Design review of the part built by this model. Coordinates are the model's own, in mm. A direction names the side the tool comes from. Coordinates: 2 decimals unless noted, no trailing zeros. Order: outer loops, then holes, each group sorted by start corner. A loop starts at its lowest first (then second) coordinate and runs counter-clockwise, first axis right, second up. Notation, with made-up numbers: M 89,55.25 L 122,55.25 A21 cw 122,83.25 Z; hole C -13,82.5 d10. An arc over 180 degrees is marked long. Use CSV: the item, a comma, the result in double quotes.
Autodesk Inventor part; units mm, degrees
ref_plane "YZ Plane" through (0, 0, 0) normal (1, 0, 0) x (0, 1, 0)
ref_plane "XZ Plane" through (0, 0, 0) normal (0, 1, 0) x (-1, 0, 0)
ref_plane "XY Plane" through (0, 0, 0) normal (0, 0, 1) x (1, 0, 0)
sketch "スケッチ1" plane through (0, 0, 0) normal (0, 0, 1) x (1, 0, 0)
  line L0 (0, 0) -> (65, 0)
  line L1 (65, 0) -> (65, 56)
  line L2 (65, 56) -> (0, 56)
  line L3 (0, 56) -> (0, 0)
  dimension "d0" = 56
  dimension "d1" = 65
extrude "押し出し1" add sketch "スケッチ1" along normal blind 1.5
sketch "スケッチ2" plane through (0, 0, 1.5) normal (0, 0, 1) x (1, 0, 0)
  line L0 (0, 0) -> (65, 0)
  line L1 (65, 0) -> (65, 56)
  line L2 (65, 56) -> (0, 56)
  line L3 (0, 56) -> (0, 0)
  line L4 (3.5, 52.5) -> (61.5, 52.5)
  line L5 (61.5, 52.5) -> (61.5, 3.5)
  line L6 (61.5, 3.5) -> (3.5, 3.5)
  line L7 (3.5, 3.5) -> (3.5, 52.5)
  dimension "d4" = 3.5
hole "穴1" at (61.5, 52.5, 1.5) at (61.5, 3.5, 1.5) at (3.5, 3.5, 1.5) at (3.5, 52.5, 1.5) direction (0, 0, -1) diameter 2.6 end through all
fillet "フィレット1" radius 3 4 edges at (0, 56, 0.75) (65, 56, 0.75) (65, 0, 0.75) (0, 0, 0.75)
sketch "スケッチ3" plane through (0, 0, 1.5) normal (0, 0, 1) x (1, 0, 0)
  arc A0 (0, 3) -> (3, 0) centre (3, 3) ccw
  line L0 (3, 0) -> (62, 0)
  arc A1 (62, 0) -> (65, 3) centre (62, 3) ccw
  line L1 (65, 3) -> (65, 53)
  arc A2 (65, 53) -> (62, 56) centre (62, 53) ccw
  line L2 (62, 56) -> (3, 56)
  arc A3 (3, 56) -> (0, 53) centre (3, 53) ccw
  line L3 (0, 53) -> (0, 3)
  circle A4 centre (3.5, 3.5) radius 1.3
  circle A5 centre (61.5, 52.5) radius 1.3
  circle A6 centre (61.5, 3.5) radius 1.3
  circle A7 centre (3.5, 52.5) radius 1.3
  line L4 (63.3, 30.32) -> (53.14, 30.32)
  line L5 (53.14, 30.32) -> (53.14, 10)
  line L6 (53.14, 10) -> (63.3, 10)
  line L7 (63.3, 10) -> (63.3, 30.32)
  point P0 (0, 0)
  dimension "d13" = 20.32
  dimension "d14" = 10.16
  dimension "d23" = 1.7
  dimension "d24" = 10
extrude "押し出し2" cut sketch "スケッチ3" against normal through all contours L7 L6 L5 L4
sketch "スケッチ4" plane through (0, 0, 1.5) normal (0, 0, 1) x (1, 0, 0)
  line L0 (53.14, 10) -> (53.14, 30.32)
  line L1 (53.14, 30.32) -> (63.3, 30.32)
  line L2 (63.3, 30.32) -> (63.3, 10)
  line L3 (63.3, 10) -> (53.14, 10)
  arc A0 (0, 3) -> (3, 0) centre (3, 3) ccw
  line L4 (3, 0) -> (62, 0)
  arc A1 (62, 0) -> (65, 3) centre (62, 3) ccw
  line L5 (65, 3) -> (65, 53)
  arc A2 (65, 53) -> (62, 56) centre (62, 53) ccw
  line L6 (62, 56) -> (3, 56)
  arc A3 (3, 56) -> (0, 53) centre (3, 53) ccw
  line L7 (0, 53) -> (0, 3)
  circle A4 centre (3.5, 3.5) radius 1.3
  circle A5 centre (61.5, 52.5) radius 1.3
  circle A6 centre (61.5, 3.5) radius 1.3
  circle A7 centre (3.5, 52.5) radius 1.3
  line L8 (57.9, 1) -> (7.1, 1)
  line L9 (7.1, 1) -> (7.1, 6.08)
  line L10 (7.1, 6.08) -> (57.9, 6.08)
  line L11 (57.9, 6.08) -> (57.9, 1)
  point P0 (0, 0)
  dimension "d17" = 5.08
  dimension "d18" = 1
  dimension "d21" = 7.1
  dimension "d22" = 50.8
extrude "押し出し3" cut sketch "スケッチ4" against normal through all contours L8 L9 L10 L11
sketch "スケッチ5" plane through (0, 0, 1.5) normal (0, 0, 1) x (1, 0, 0)
  line L0 (57.9, 6.08) -> (57.9, 1)
  line L1 (57.9, 1) -> (7.1, 1)
  line L2 (7.1, 1) -> (7.1, 6.08)
  line L3 (7.1, 6.08) -> (57.9, 6.08)
  line L4 (53.14, 10) -> (53.14, 30.32)
  line L5 (53.14, 30.32) -> (63.3, 30.32)
  line L6 (63.3, 30.32) -> (63.3, 10)
  line L7 (63.3, 10) -> (53.14, 10)
  arc A0 (0, 3) -> (3, 0) centre (3, 3) ccw
  line L8 (3, 0) -> (62, 0)
  arc A1 (62, 0) -> (65, 3) centre (62, 3) ccw
  line L9 (65, 3) -> (65, 53)
  arc A2 (65, 53) -> (62, 56) centre (62, 53) ccw
  line L10 (62, 56) -> (3, 56)
  arc A3 (3, 56) -> (0, 53) centre (3, 53) ccw
  line L11 (0, 53) -> (0, 3)
  circle A4 centre (3.5, 3.5) radius 1.3
  circle A5 centre (61.5, 52.5) radius 1.3
  circle A6 centre (61.5, 3.5) radius 1.3
  circle A7 centre (3.5, 52.5) radius 1.3
  line L12 (58.5, 56) -> (44.5, 56)
  line L13 (44.5, 56) -> (44.5, 52)
  line L14 (44.5, 52) -> (58.5, 52)
  line L15 (58.5, 52) -> (58.5, 56)
  line L16 (17.5, 44) -> (44.5, 44)
  line L17 (44.5, 44) -> (44.5, 56)
  line L18 (44.5, 56) -> (17.5, 56)
  line L19 (17.5, 56) -> (17.5, 44)
  point P0 (0, 0)
  dimension "d25" = 3
  dimension "d26" = 4
  dimension "d27" = 14
  dimension "d28" = 27
  dimension "d29" = 12
extrude "押し出し4" cut sketch "スケッチ5" against normal through all contours L10 L13 L17 L16 L19 | L10 L15 L14 L13
fillet "フィレット2" radius 1 3 edges at (58.5, 56, 0.75) (44.5, 52, 0.75) (17.5, 56, 0.75)
fillet "フィレット2" radius 1 3 edges at (58.5, 52, 0.75) (44.5, 44, 0.75) (17.5, 44, 0.75)
fillet "フィレット3" radius 0.5 8 edges at (57.9, 1, 0.75) (57.9, 6.08, 0.75) (63.3, 10, 0.75) (53.14, 10, 0.75) (53.14, 30.32, 0.75) (63.3, 30.32, 0.75) (7.1, 1, 0.75) (7.1, 6.08, 0.75)
properties part number "ボードガード" material "アルミニウム 6061"
(1) Add section D-D on z = 0.65. Give the number of separate pieces and of enclosed holes in the cut face, and give its area (3 significant figures).
The answers:
separate pieces,"1"
enclosed holes,"6"
area,"2,770 mm2"
(2) For faces 1 (the face through (64.1, 0.86, 0.76)), 2 (the face through (32, 6.08, 1)), 3 (the face through (31, 44, 1)), list the 3-axis set-ups (+Z, -Z, +X, -X, +Y, -Y) from which the entire face can be reached by the end or side of a thin tool; tool diameter is ignored.
The answers:
face 1,"+Z, -Z, +X, -Y"
face 2,"+Z, -Z"
face 3,"+Z, -Z, +Y"
(3) Add section B-B on y = 24.5. State the section outline as (x, z) points, and give its area (3 significant figures).
The answers:
outline,"M 0,0 L 53.14,0 L 53.14,1.5 L 0,1.5 Z; M 63.3,0 L 65,0 L 65,1.5 L 63.3,1.5 Z"
area,"82.3 mm2"
(4) Add section A-A on x = 54.5. State the section outline as (y, z) points.
The answers:
outline,"M 0,0 L 1,0 L 1,1.5 L 0,1.5 Z; M 6.08,0 L 10,0 L 10,1.5 L 6.08,1.5 Z; M 30.32,0 L 52,0 L 52,1.5 L 30.32,1.5 Z"
(5) Wall thickness on probe 1 along Y at (x, z) = (3.5, 1.05); probe 2 along Y at (x, z) = (61.5, 0.5); probe 3 along X at (y, z) = (3.5, 0.85): over which ranges is each line inside the solid? List them lowest first.
The answers:
probe 1,"y = 0 to 2.2, 4.8 to 51.2, 53.8 to 56"
probe 2,"y = 0 to 2.2, 4.8 to 10, 30.32 to 51.2, 53.8 to 56"
probe 3,"x = 0 to 2.2, 4.8 to 7.1, 57.9 to 60.2, 62.8 to 65"
(6) The part is to be moulded in two halves that separate along Y. For faces 4 (the face through (58, 30.32, 1)), 5 (the face through (0.86, 0.9, 0.76)), 6 (the face through (0, 28, 1)), say which applies: pulls with the +Y half, pulls with the -Y half, needs draft (parallel to the pull), parting line crosses it, or undercut.
The answers:
face 4,"undercut"
face 5,"pulls with the -Y half"
face 6,"needs draft"
(7) Clearance check with flat-ended pins moving along their axes: P1, Ø0.8, axis at x = 40.5, z = 0.5, coming from the +Y side; P2, Ø2, axis at x = 3.5, y = 52.5, coming from the -Z side. State where each tip first meets the part, or that it passes through.
The answers:
P1,"stops at y = 44"
P2,"passes through"
(8) Add section C-C on x = 38. State the section outline as (y, z) points, and give its area (3 significant figures).
The answers:
outline,"M 0,0 L 1,0 L 1,1.5 L 0,1.5 Z; M 6.08,0 L 44,0 L 44,1.5 L 6.08,1.5 Z"
area,"58.4 mm2"
